```python
from build123d import *

# Parameters (mm, degrees)
BOSS_EXTRUDE1_DEPTH   = 3.175
SKETCH2_R             = 8.255
CUT_EXTRUDE1_DEPTH    = 102.488814162
F_8_CLEARANCE_HOLE1_D = 4.3053
CIRPATTERN1_COUNT     = 6
FILLET1_R             = 3.175
CUT_EXTRUDE2_DEPTH    = 102.488814162
FILLET2_R             = 6.35


with BuildPart() as part:
    # Sketch1 → Boss-Extrude1 (new, symmetric)
    with BuildSketch(Plane(origin=(0, 0, 0), x_dir=(0, 0, -1), z_dir=(1, 0, 0))):
        with BuildLine():
            Line((0, -34.925), (0, 34.925))
            Line((0, 34.925), (9.525, 34.925))
            Line((9.525, 34.925), (79.8090967, -16.361371494))
            ThreePointArc((79.8090967, -16.361371494), (85.714272022, -40.075816614), (63.420756295, -50.088067084))
            Line((63.420756295, -50.088067084), (9.525, -34.925))
            Line((9.525, -34.925), (0, -34.925))
        make_face()
    extrude(amount=BOSS_EXTRUDE1_DEPTH, both=True)

    # Sketch2 → Cut-Extrude1 (cut, through all)
    with BuildSketch(Plane(origin=(3.175, 0, 0), x_dir=(0, 0, -1), z_dir=(1, 0, 0))):
        with Locations((68.58, -31.75)):
            Circle(SKETCH2_R)
    extrude(amount=-CUT_EXTRUDE1_DEPTH, mode=Mode.SUBTRACT)

    # #8 Clearance Hole1 (through all)
    with Locations(Plane(origin=(3.175, 0, 0), x_dir=(0, 0, -1), z_dir=(1, 0, 0))):
        with Locations((4.7625, 0), (4.7625, 28.575), (4.7625, -28.575)):
            Hole(F_8_CLEARANCE_HOLE1_D / 2)

    # Sketch6 → #4 Clearance Hole1 (revolve, cut)
    with BuildSketch(Plane(origin=(3.175, -16.51, -68.58), x_dir=(0, 0, -1), z_dir=(0, 1, 0))):
        Polygon((0, 0), (0, 7.235187864), (1.4732, 6.35), (1.4732, 0), align=None)
    f_4_clearance_hole1 = revolve(axis=Axis((9.525, -16.51, -68.58), (-1, 0, 0)), mode=Mode.SUBTRACT)

    # CirPattern1: #4 Clearance Hole1 ×6 about axis
    cirpattern1_axis = Axis((0, -31.75, -68.58), (1, 0, 0))
    for i in range(1, CIRPATTERN1_COUNT):
        add(f_4_clearance_hole1.rotate(cirpattern1_axis, i * 360 / CIRPATTERN1_COUNT), mode=Mode.SUBTRACT)

    # Fillet1
    fillet1_edges = [part.edges().sort_by_distance(p)[0] for p in [
        (0, 34.925, -9.525),
        (0, -34.925, -9.525),
    ]]
    fillet(fillet1_edges, radius=FILLET1_R)

    # Sketch8 → Cut-Extrude2 (cut, through all)
    with BuildSketch(Plane(origin=(3.175, 0, 0), x_dir=(0, 0, -1), z_dir=(1, 0, 0))):
        with BuildLine():
            Line((12.7, -25.923470533), (12.7, 20.816944046))
            Line((12.7, 20.816944046), (57.973509635, -12.219178534))
            ThreePointArc((57.973509635, -12.219178534), (48.590015975, -22.036547283), (46.67035819, -35.480713171))
            Line((46.67035819, -35.480713171), (12.7, -25.923470533))
        make_face()
    extrude(amount=-CUT_EXTRUDE2_DEPTH, mode=Mode.SUBTRACT)

    # Fillet2
    fillet2_edges = [part.edges().sort_by_distance(p)[0] for p in [
        (0, -35.480713171, -46.67035819),
        (0, -25.923470533, -12.7),
        (0, 20.816944046, -12.7),
        (0, -12.219178534, -57.973509635),
    ]]
    fillet(fillet2_edges, radius=FILLET2_R)


solid = part.part
```
Input: part model. Units: mm. Frame: model coordinates. A direction names the side the tool comes from. Coordinates: 2 decimals unless noted, no trailing zeros. Loops run counter-clockwise (first coordinate to the right, second up) from the corner with the lowest first, then second, coordinate; pieces in that order, holes last.
Q1. Section A-A, the plane z = -68.58. Return the cut outline in (x, y) (3 decimals), and give its area (3 significant figures).
Results are:
outline: (-3.175, -50.8) - (3.175, -50.8) - (3.175, -48.463) - (-3.175, -48.463) - close; (-3.175, -45.517) - (3.175, -45.517) - (3.175, -40.005) - (-3.175, -40.005) - close; (-3.175, -23.495) - (3.175, -23.495) - (3.175, -17.983) - (-3.175, -17.983) - close; (-3.175, -15.037) - (3.175, -15.037) - (3.175, -8.167) - (-3.175, -8.167) - close
area: 128 mm2
Q2. Section B-B, the plane y = -46.99. Return the cut outline in (x, z) (3 decimals).
Results are:
outline: (-3.175, -80.01) - (3.175, -80.01) - (3.175, -70.053) - (-3.175, -70.053) - close; (-3.175, -67.107) - (3.175, -67.107) - (3.175, -52.409) - (-3.175, -52.409) - close
Q3. Line query: line 1 along Y through (x, z) = (-0.75, -4.5) (3 decimals); line 2 along Y through (x, z) = (-1, -68); line 3 along Y through (x, z) = (1, -76). Output: solid intervals per line, ascending.
Results are:
line 1: y = -34.925 to -30.712, -26.438 to -2.137, 2.137 to 26.438, 30.712 to 34.925
line 2: y = -50.79 to -48.34, -45.64 to -39.98, -23.52 to -17.86, -15.16 to -7.74
line 3: y = -49.3 to -35.37, -28.13 to -13.58
Q4. Set-up query: faces 1 (the cylindrical face through (-0.044, 34.773, -9.461)), 2 (the flat face through (0.044, 3.213, -36.825)). Return all of +Z, -Z, +X, -X, +Y, -Y with unobstructed straight access to the full face (end or side cutting, diameter ignored); none if empty.
Results are:
face 1: -Z, +X, -X, +Y
face 2: +X, -X
Q5. Mould query, pull axis Y, two halves, no side actions, for faces 3 (the cylindrical face through (0.044, -15.946, -69.941)), 4 (the flat face through (-3.175, 2, -44)), 5 (the cylindrical face through (-0.044, 26.474, -5.229)), 6 (the flat face through (0, 34.925, -4)). Classes: +Y half, -Y half, draft (parallel to the pull), parting line (faces both ways), or undercut.
Results are:
face 3: undercut
face 4: draft
face 5: undercut
face 6: +Y half
Q6. Section C-C, the plane x = 1.25. Give the number of separate pieces and of enclosed holes in the cut face, and give its area (3 significant figures).
Results are:
separate pieces: 1
enclosed holes: 11
area: 2,930 mm2
Q7. Contact query for flat-ended pins moving along their axis: pin 1 (1.5 mm diameter, centred on x = 2, y = -37.5, fed in from -Z); pin 2 (1.9 mm diameter, centred on x = -1, y = -11.5, fed in from -Z). Output: stop coordinate, or through.
Results are:
pin 1: stops at z = -86.96
pin 2: stops at z = -74.45
Q8. Section D-D, the plane z = -35. Return the cut outline in (x, y) (3 decimals).
Results are:
outline: (-3.175, -42.092) - (3.175, -42.092) - (3.175, -32.197) - (-3.175, -32.197) - close; (-3.175, 4.545) - (3.175, 4.545) - (3.175, 16.336) - (-3.175, 16.336) - close
